Read the model definition and answer for the solid it produces. Units are mm, in the model's axes. A direction names the side the tool comes from. Give positions to 0.01 mm unless a question says otherwise; leave off trailing zeros. Loops run counter-clockwise (first coordinate to the right, second up) from the corner with the lowest first, then second, coordinate; pieces in that order, holes last. Notation, with made-up numbers: M 55,41.5 L 105,41.5 A12 ccw 105,46.5 Z; hole C 50.25,-5.75 d9. An arc over 180 degrees is marked long. Return JSON: item names as keys, results as strings. Group by question number.
```python
from build123d import *

# Parameters (mm, degrees)
F0_W          = 25.4
F0_H          = 15.875
F1_DEPTH      = 69.05625
F1_DEPTH_BACK = 69.05625
F2_R          = 4.7625
F3_DEPTH      = 15.876
F4_R          = 3.175
F5_DEPTH      = 25.4


with BuildPart() as f1:
    # F0 (on Front) → F1 (new body, two sides)
    with BuildSketch(Plane.XZ) as f1_sk:
        Rectangle(F0_W, F0_H)
    extrude(amount=-F1_DEPTH)
    extrude(f1_sk.sketch, amount=F1_DEPTH_BACK)

    # F2 (on face) → F3 (cut, through all)
    with BuildSketch(Plane.XY.offset(7.9375)):
        with Locations((0, -53.18125)):
            Circle(F2_R)
    extrude(amount=-F3_DEPTH, mode=Mode.SUBTRACT)

    # F4 (on face) → F5 (cut)
    with BuildSketch(Plane.XZ.offset(69.05625)):
        Circle(F4_R)
    extrude(amount=-F5_DEPTH, mode=Mode.SUBTRACT)


solid = f1.part
```
1. The mould has two halves that part along X. Classify faces 3 (the cylindrical face through (-4.758, -52.972, 0.111)), 4 (the flat face through (-12.7, 1, 0)), 5 (the flat face through (0, 1, 7.938)): +X half, -X half, draft (parallel to the pull), parting line (faces both ways), or undercut.
2. Find section C-C (z = 5). Write down the section's boundary in (x, y) (1 decimal).
3. A flat-ended cylindrical pin translates along its axis: P1, Ø3, axis at x = 1, z = 0, coming from the -Y side. Find the tip coordinate at first contact, or state that the pin passes through.
4. Find section B-B (z = 0). Write down the section's boundary in (x, y) (1 decimal).
5. For faces 1 (the cylindrical face through (-3.17, -62.98, 0.14)), 2 (the flat face through (0, 1, -7.938)), determine the directions among +Z, -Z, +X, -X, +Y, -Y from which every point of the face is accessible in a straight line to the end or side of a thin tool.
6. Find section A-A (x = 0). Write down the section's boundary in (y, z) (1 decimal).
7. Straight lines are drawn through the part: line 1 along Y through (x, z) = (0, 3.75); line 2 along X through (y, z) = (-47.5, 0) (3 decimals); line 3 along Z through (x, y) = (0, -48.3) (1 decimal). For each, find the intervals that lie inside material, in ascending order.
Result:
{
 "1": {"face 3": "undercut", "face 4": "-X half", "face 5": "draft"},
 "2": {"outline": "M -12.7,-69.1 L 12.7,-69.1 L 12.7,69.1 L -12.7,69.1 Z; hole C 0,-53.2 d9.5"},
 "3": {"P1": "stops at y = -43.66"},
 "4": {"outline": "M -12.7,-69.1 L -3.2,-69.1 L -3.2,-56.7 A4.8 cw -3.2,-49.6 L -3.2,-43.7 L 3.2,-43.7 L 3.2,-49.6 A4.8 cw 3.2,-56.7 L 3.2,-69.1 L 12.7,-69.1 L 12.7,69.1 L -12.7,69.1 Z"},
 "5": {"face 1": "-Y", "face 2": "-Z, +X, -X, +Y, -Y"},
 "6": {"outline": "M -69.1,-7.9 L -57.9,-7.9 L -57.9,-3.2 L -69.1,-3.2 Z; M -69.1,3.2 L -57.9,3.2 L -57.9,7.9 L -69.1,7.9 Z; M -48.4,-7.9 L 69.1,-7.9 L 69.1,7.9 L -48.4,7.9 L -48.4,3.2 L -43.7,3.2 L -43.7,-3.2 L -48.4,-3.2 Z"},
 "7": {"line 1": "y = -69.06 to -57.94, -48.42 to 69.06", "line 2": "x = -12.7 to -3.175, 3.175 to 12.7", "line 3": "z = -7.9 to -3.2, 3.2 to 7.9"}
}
